Could you check a few things on this drawing? It's one solid part, dimensions in mm from its lowest x, y, z. A direction names the side the tool comes from. Give positions to 0.01 mm unless a question says otherwise; leave off trailing zeros. Loops run counter-clockwise (first coordinate to the right, second up) from the corner with the lowest first, then second, coordinate; pieces in that order, holes last.
Q1. Thinking about a two-plate mould opening in Y: for the marked faces 1, 2, 3 and 4, which applies, pulls with the +Y half, pulls with the -Y half, needs draft (parallel to the pull), parting line crosses it, or undercut?
Q2. Suppose I cut it at D-D (z = 8.75). List the corners of the cut face in (x, y) for me.
Q3. I'm going to push flat-ended pins straight in: P1, Ø4, axis at x = 8.5, y = 4, coming from the +Z side; P2, Ø4, axis at x = 21.5, z = 4.5, coming from the -Y side; P3, Ø5, axis at x = 9.5, z = 2.5, coming from the -Y side. Where does each tip first touch, or does it pass through?
Q4. Suppose I cut it at B-B (z = 3.5). List the corners of the cut face in (x, y) for me, and give its area (3 significant figures).
Q5. Suppose I cut it at A-A (y = 22). List the corners of the cut face in (x, z) for me (1 decimal).
Q6. I need wall thicknesses on probe 1 along X at (y, z) = (16, 8.75); probe 2 along Z at (x, y) = (14.5, 1); probe 3 along X at (y, z) = (16, 1.75). Which ranges of each line are inside material? Lowest first, please.
Q7. For the marked faces 5 and 6, which set-ups out of +Z, -Z, +X, -X, +Y, -Y let a thin tool reach every point of the face, with its end or its side?
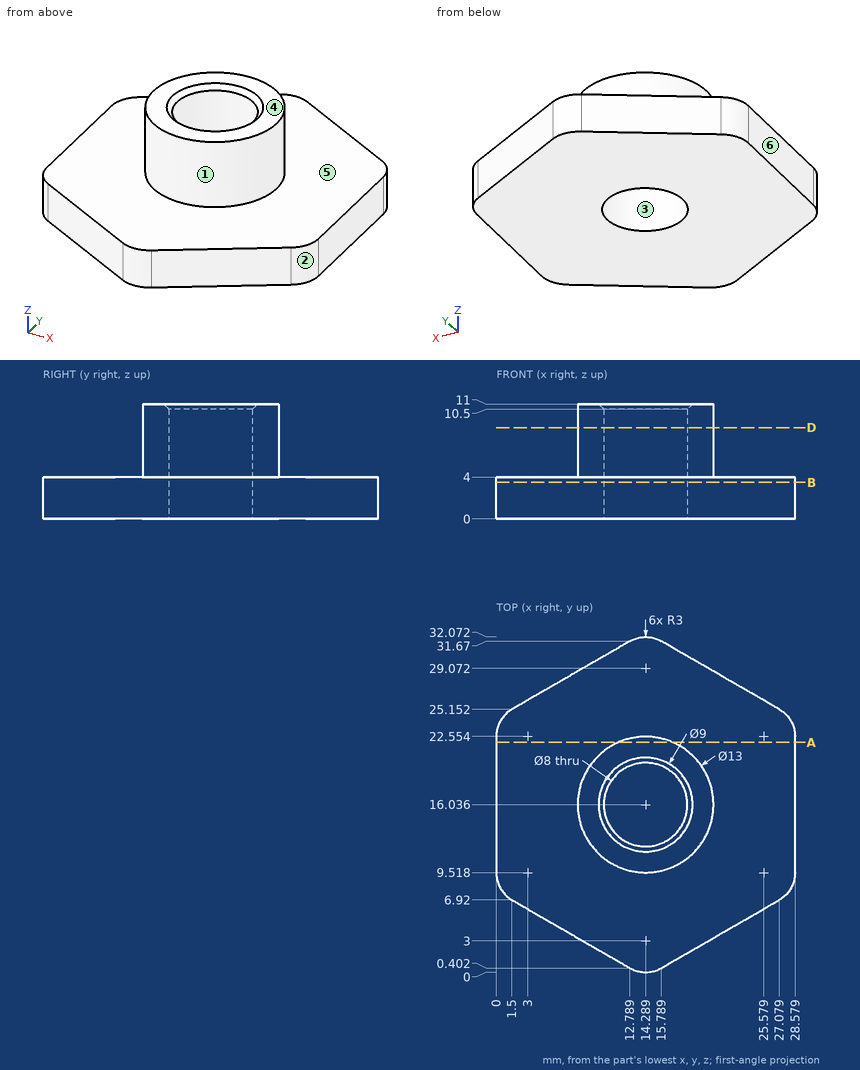
Solutions:
1. face 1: parting line crosses it
1. face 2: pulls with the -Y half
1. face 3: undercut
1. face 4: needs draft
2. outline: circle Ø13 at (14.29, 16.04); hole circle Ø8 at (14.29, 16.04)
3. P1: stops at z = 4
3. P2: stops at y = 2.58
3. P3: stops at y = 0.86
4. outline: (0, 9.52) arc R3 ccw to (1.5, 6.92) - (12.79, 0.4) arc R3 ccw to (15.79, 0.4) - (27.08, 6.92) arc R3 ccw to (28.58, 9.52) - (28.58, 22.55) arc R3 ccw to (27.08, 25.15) - (15.79, 31.67) arc R3 ccw to (12.79, 31.67) - (1.5, 25.15) arc R3 ccw to (0, 22.55) - close; hole circle Ø8 at (14.29, 16.04)
4. area: 654 mm2
5. outline: (0, 0) - (28.6, 0) - (28.6, 4) - (16.9, 4) - (16.9, 11) - (11.7, 11) - (11.7, 4) - (0, 4) - close
6. probe 1: x = 7.79 to 10.29, 18.29 to 20.79
6. probe 2: z = 0 to 4
6. probe 3: x = 0 to 10.29, 18.29 to 28.58
7. face 5: +Z
7. face 6: +Z, -Z, -X, +Y, -Y
